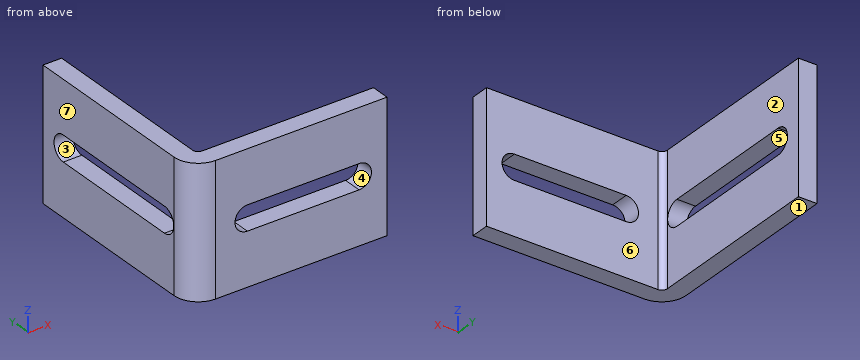
from build123d import *

# Parameters (mm, degrees)
CROQUIS1_W                    = 70
CROQUIS1_H                    = 110
SALIENTE_EXTRUIR1_DEPTH       = 7.9375
CROQUIS2_W                    = 97.0625
CROQUIS2_H                    = 70
SALIENTE_EXTRUIR2_DEPTH       = 7.9375
CONVERTIR_S_LIDO1_START       = -22.0625
CONVERTIR_S_LIDO1_OUTLINE_W   = 97.0625
CONVERTIR_S_LIDO1_OUTLINE_H   = 70
CONVERTIR_S_LIDO1_DEPTH       = 5.0625
CONVERTIR_S_LIDO1_START_2     = -18.37306
CONVERTIR_S_LIDO1_2_OUTLINE_W = 2.0625
CONVERTIR_S_LIDO1_2_OUTLINE_H = 28.16517088
CONVERTIR_S_LIDO1_2_DEPTH     = 98.37306
CONVERTIR_S_LIDO1_START_3     = 65
CONVERTIR_S_LIDO1_3_OUTLINE_W = 2.0625
CONVERTIR_S_LIDO1_3_OUTLINE_H = 13.66965824
CONVERTIR_S_LIDO1_3_DEPTH     = 15
CONVERTIR_S_LIDO1_4_OUTLINE_W = 2.0625
CONVERTIR_S_LIDO1_4_OUTLINE_H = 13.66965824
CONVERTIR_S_LIDO1_4_DEPTH     = 8.37306
CONVERTIR_S_LIDO1_START_4     = 13
CONVERTIR_S_LIDO1_5_OUTLINE_W = 3
CONVERTIR_S_LIDO1_5_OUTLINE_H = 70
CONVERTIR_S_LIDO1_5_DEPTH     = 92
CONVERTIR_S_LIDO1_START_5     = 7.9375
CONVERTIR_S_LIDO1_6_DEPTH     = 2.0625
CONVERTIR_S_LIDO1_START_6     = -35
CONVERTIR_S_LIDO1_7_DEPTH     = 70


with BuildPart() as part:
    # Croquis1 → Saliente-Extruir1 (new body)
    with BuildSketch(Plane(origin=(0, 0, 0), x_dir=(0, 0, -1), z_dir=(1, 0, 0))):
        with Locations((0, 25)):
            Rectangle(CROQUIS1_W, CROQUIS1_H)
        with BuildLine():
            Line((6.83482912, 65), (6.83482912, -10))
            ThreePointArc((6.83482912, -10), (0, -16.83482912), (-6.83482912, -10))
            Line((-6.83482912, -10), (-6.83482912, 65))
            ThreePointArc((-6.83482912, 65), (0, 71.83482912), (6.83482912, 65))
        make_face(mode=Mode.SUBTRACT)
    extrude(amount=SALIENTE_EXTRUIR1_DEPTH)

    # Croquis2 → Saliente-Extruir2 (add)
    with BuildSketch(Plane.XZ.offset(30)):
        with Locations((56.46875, 0)):
            Rectangle(CROQUIS2_W, CROQUIS2_H)
        with BuildLine():
            ThreePointArc((30, -6.640349162), (23.359650838, 0), (30, 6.640349162))
            Line((30, 6.640349162), (90, 6.640349162))
            ThreePointArc((90, 6.640349162), (96.640349162, 0), (90, -6.640349162))
            Line((90, -6.640349162), (30, -6.640349162))
        make_face(mode=Mode.SUBTRACT)
    extrude(amount=-SALIENTE_EXTRUIR2_DEPTH)

    # Convertir-Sólido1: read off the stored shape, not the designer's step
    # Convertir-Sólido1 outline → Convertir-Sólido1 (add)
    with BuildSketch(Plane(origin=(0, 0, 0), x_dir=(1, 0, 0), z_dir=(0, 1, 0)).offset(CONVERTIR_S_LIDO1_START)):
        with Locations((56.46875, 0)):
            Rectangle(CONVERTIR_S_LIDO1_OUTLINE_W, CONVERTIR_S_LIDO1_OUTLINE_H)
        with BuildLine():
            Line((90, -6.640349162), (30, -6.640349162))
            ThreePointArc((30, -6.640349162), (23.359650838, 0), (30, 6.640349162))
            Line((30, 6.640349162), (90, 6.640349162))
            ThreePointArc((90, 6.640349162), (96.640349162, 0), (90, -6.640349162))
        make_face(mode=Mode.SUBTRACT)
    extrude(amount=CONVERTIR_S_LIDO1_DEPTH)

    # Convertir-S_lido1 2 outline → Convertir-S_lido1 2 (add)
    with BuildSketch(Plane(origin=(0, 0, 0), x_dir=(1, 0, 0), z_dir=(0, 1, 0)).offset(CONVERTIR_S_LIDO1_START_2)):
        with Locations((8.96875, 20.91741456)):
            Rectangle(CONVERTIR_S_LIDO1_2_OUTLINE_W, CONVERTIR_S_LIDO1_2_OUTLINE_H)
        with Locations((8.96875, -20.91741456)):
            Rectangle(CONVERTIR_S_LIDO1_2_OUTLINE_W, CONVERTIR_S_LIDO1_2_OUTLINE_H)
    extrude(amount=CONVERTIR_S_LIDO1_2_DEPTH)

    # Convertir-S_lido1 3 outline → Convertir-S_lido1 3 (add)
    with BuildSketch(Plane(origin=(0, 0, 0), x_dir=(1, 0, 0), z_dir=(0, 1, 0)).offset(CONVERTIR_S_LIDO1_START_3)):
        with Locations((8.96875, 0)):
            Rectangle(CONVERTIR_S_LIDO1_3_OUTLINE_W, CONVERTIR_S_LIDO1_3_OUTLINE_H)
    extrude(amount=CONVERTIR_S_LIDO1_3_DEPTH)

    # Convertir-S_lido1 4 outline → Convertir-S_lido1 4 (add)
    with BuildSketch(Plane(origin=(0, 0, 0), x_dir=(1, 0, 0), z_dir=(0, 1, 0)).offset(CONVERTIR_S_LIDO1_START_2)):
        with Locations((8.96875, 0)):
            Rectangle(CONVERTIR_S_LIDO1_4_OUTLINE_W, CONVERTIR_S_LIDO1_4_OUTLINE_H)
    extrude(amount=CONVERTIR_S_LIDO1_4_DEPTH)

    # Convertir-S_lido1 5 outline → Convertir-S_lido1 5 (cut)
    with BuildSketch(Plane.YZ.offset(CONVERTIR_S_LIDO1_START_4)):
        with Locations((-18.5, 0)):
            Rectangle(CONVERTIR_S_LIDO1_5_OUTLINE_W, CONVERTIR_S_LIDO1_5_OUTLINE_H)
    extrude(amount=CONVERTIR_S_LIDO1_5_DEPTH, mode=Mode.SUBTRACT)

    # Convertir-S_lido1 6 outline → Convertir-S_lido1 6 (cut)
    with BuildSketch(Plane.YZ.offset(CONVERTIR_S_LIDO1_START_5)):
        with BuildLine():
            Line((65, 6.83482912), (65, -6.83482912))
            ThreePointArc((65, -6.83482912), (71.83482912, 0), (65, 6.83482912))
        make_face()
        with BuildLine():
            Line((-10, -6.83482912), (-10, 6.83482912))
            ThreePointArc((-10, 6.83482912), (-16.83482912, 0), (-10, -6.83482912))
        make_face()
    extrude(amount=CONVERTIR_S_LIDO1_6_DEPTH, mode=Mode.SUBTRACT)

    # Convertir-S_lido1 7 outline → Convertir-S_lido1 7 (cut)
    with BuildSketch(Plane.XY.offset(CONVERTIR_S_LIDO1_START_6)):
        with BuildLine():
            Line((0, -30), (13, -30))
            ThreePointArc((13, -30), (3.807611845, -26.192388155), (0, -17))
            Line((0, -17), (0, -30))
        make_face()
        with BuildLine():
            ThreePointArc((10, -17), (10.878679656, -19.121320344), (13, -20))
            Line((13, -20), (13, -17))
            Line((13, -17), (10, -17))
        make_face()
    extrude(amount=CONVERTIR_S_LIDO1_7_DEPTH, mode=Mode.SUBTRACT)


solid = part.part
Part model, mm, in its own coordinate system. Face numbers are marked on the shaded views. A direction names the side the tool comes from. Round coordinates to 2 decimals unless told otherwise and drop trailing zeros. Write each loop counter-clockwise with the first axis right and the second up, starting at its lowest first coordinate (ties: lowest second). Pieces come first, ordered by that corner, then holes. Notation, with made-up numbers: M 83.5,5 L 124.5,5 A9 cw 124.5,22 Z; hole C 53,-12.75 d2. An arc over 180 degrees is marked long. Return JSON: item names as keys, results as strings. Group by question number.
(1) Drill centre lines: probe 1 along X at (y, z) = (54.5, -8); probe 2 along Y at (x, z) = (16.5, -14); probe 3 along Z at (x, y) = (28, -23.5). Where is each one in solid material? Low to high.
(2) Two-plate mould, pull along Z, no slides. Class the marked faces 1, 2, 3 and 4: +Z half, -Z half, draft (parallel to the pull), parting line (faces both ways), or undercut.
(3) Saw through at B-B on z = 0. Write the cut outline in (x, y).
(4) Saw through at A-A on x = 76. Write the cut outline in (y, z), then the cut area to 3 significant figures.
(5) Which spindle directions (+Z, -Z, +X, -X, +Y, -Y) get a long thin tool onto all of the face, cutting with end or side? Do the marked faces 5, 6 and 7. Say none if no direction does.
(6) Saw through at D-D on y = -22. Write the cut outline in (x, z), then the cut area to 3 significant figures.
(7) Saw through at C-C on y = 35. Write the cut outline in (x, z).
(8) Pin check, flat tips, straight feed: pin 1 Ø5 at (x, y) = (54, -16) entering from +Z; pin 2 Ø3 at (y, z) = (-5.5, -20) entering from +X; pin 3 Ø1.5 at (x, z) = (61, 22) entering from +Y. Stop position of each tip, or through.
Returned:
{
 "1": {"probe 1": "0 to 10", "probe 2": "-30 to -20", "probe 3": "-35 to -6.33, 6.33 to 35"},
 "2": {"face 1": "-Z half", "face 2": "draft", "face 3": "undercut", "face 4": "undercut"},
 "3": {"outline": "M 0,-17 A13 ccw 13,-30 L 23.36,-30 L 23.36,-20 L 13,-20 A3 cw 10,-17 L 10,-16.83 L 0,-16.83 Z; M 0,71.83 L 10,71.83 L 10,80 L 0,80 Z; M 96.64,-30 L 105,-30 L 105,-20 L 96.64,-20 Z"},
 "4": {"outline": "M -30,-35 L -20,-35 L -20,-6.64 L -30,-6.64 Z; M -30,6.64 L -20,6.64 L -20,35 L -30,35 Z", "area": "567 mm²"},
 "5": {"face 5": "+X, -X", "face 6": "+Z, -Z, +X, +Y", "face 7": "+Z, -Z, -X, +Y, -Y"},
 "6": {"outline": "M 1,-35 L 105,-35 L 105,35 L 1,35 Z; hole M 30,-6.64 L 90,-6.64 A6.64 ccw 90,6.64 L 30,6.64 A6.64 ccw Z", "area": "6,340 mm²"},
 "7": {"outline": "M 0,-35 L 10,-35 L 10,-6.83 L 0,-6.83 Z; M 0,6.83 L 10,6.83 L 10,35 L 0,35 Z"},
 "8": {"pin 1": "through", "pin 2": "x = 10", "pin 3": "y = -20"}
}
